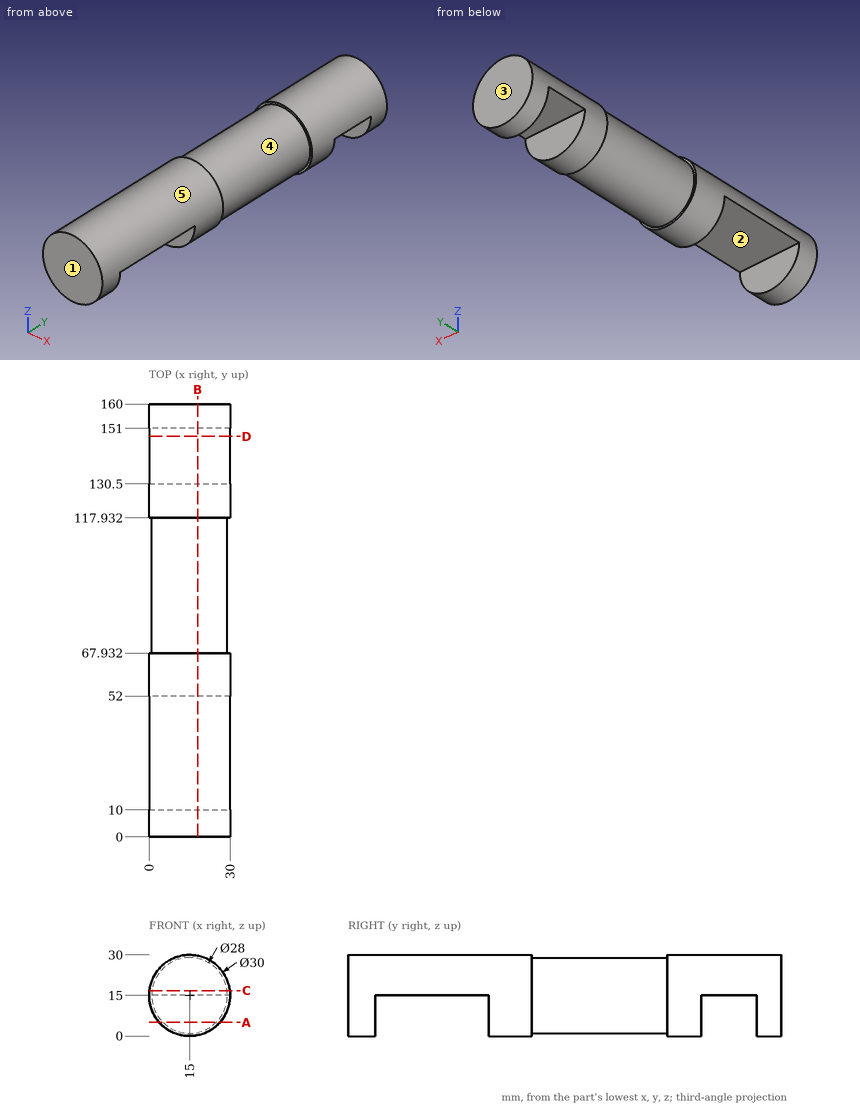
Design review of the part shown in the three views and the two pictorial views. Dimensions are in mm from the part's minimum x, y and z. A direction names the side the tool comes from. Give positions to 0.01 mm unless a question says otherwise; leave off trailing zeros. Loops run counter-clockwise (first coordinate to the right, second up) from the corner with the lowest first, then second, coordinate; pieces in that order, holes last. Notation, with made-up numbers: M 39,86.5 L 81,86.5 A31 cw 81,112.5 Z; hole C -31.75,3 d3. An arc over 180 degrees is marked long. Answer as a JSON object with one key per item and string values. Group by question number.
Q1. Add section D-D on y = 148. Give the boundary of the cut face in (x, z), and give its area (3 significant figures).
Q2. Insertion check: P1, Ø4, axis at y = 43, z = 19.5, coming from the +X side; P2, Ø1.5, axis at x = 25, y = 108, coming from the +Z side; P3, Ø5, axis at x = 4.5, y = 66.5, coming from the -Z side. Each pin has a flat end and moves straight along its axis. Give the tip position at first contact, or say it passes through.
Q3. Add section A-A on z = 5. Give the boundary of the cut face in (x, y).
Q4. For probe 1 along Y at (x, z) = (9.5, 10); probe 2 along Z at (x, y) = (14.5, 62); probe 3 along Z at (x, y) = (14.5, 19.5), list the stretches that pass through material, from the lowest coordinate up. Write a range as [from, to].
Q5. Add section B-B on x = 18. Give the boundary of the cut face in (y, z) (1 decimal).
Q6. Add section C-C on z = 16.75. Give the boundary of the cut face in (x, y), and give its area (3 significant figures).
Q7. Mouldability with a two-part tool opening along Y and no side actions: class the marked faces 3, 4 and 5 as +Y half, -Y half, draft (parallel to the pull), parting line (faces both ways), or undercut.
Q8. Tool access review of the marked faces 1 and 2: name each direction out of +Z, -Z, +X, -X, +Y, -Y from which nothing blocks a thin tool from reaching the whole face with its end or side.
Checked values:
{
 "1": {"outline": "M 0,15 L 30,15 A15 ccw Z", "area": "353 mm²"},
 "2": {"P1": "x = 29.79", "P2": "z = 25.51", "P3": "z = 2.31"},
 "3": {"outline": "M 3.82,0 L 26.18,0 L 26.18,10 L 3.82,10 Z; M 3.82,52 L 26.18,52 L 26.18,67.93 L 24.8,67.93 L 24.8,117.93 L 26.18,117.93 L 26.18,130.5 L 3.82,130.5 L 3.82,117.93 L 5.2,117.93 L 5.2,67.93 L 3.82,67.93 Z; M 3.82,151 L 26.18,151 L 26.18,160 L 3.82,160 Z"},
 "4": {"probe 1": "[0, 10], [52, 130.5], [151, 160]", "probe 2": "[0.01, 29.99]", "probe 3": "[15, 29.99]"},
 "5": {"outline": "M 0,0.3 L 10,0.3 L 10,15 L 52,15 L 52,0.3 L 67.9,0.3 L 67.9,1.3 L 117.9,1.3 L 117.9,0.3 L 130.5,0.3 L 130.5,15 L 151,15 L 151,0.3 L 160,0.3 L 160,29.7 L 117.9,29.7 L 117.9,28.7 L 67.9,28.7 L 67.9,29.7 L 0,29.7 Z"},
 "6": {"outline": "M 0.1,0 L 29.9,0 L 29.9,67.93 L 28.89,67.93 L 28.89,117.93 L 29.9,117.93 L 29.9,160 L 0.1,160 L 0.1,117.93 L 1.11,117.93 L 1.11,67.93 L 0.1,67.93 Z", "area": "4,670 mm²"},
 "7": {"face 3": "+Y half", "face 4": "undercut", "face 5": "draft"},
 "8": {"face 1": "+Z, -Z, +X, -X, -Y", "face 2": "-Z, +X, -X"}
}
